For this review, take the finished solid that the model builds, in its own axes (mm). Round coordinates to 2 decimals unless told otherwise and drop trailing zeros. Loops run counter-clockwise (first coordinate to the right, second up) from the corner with the lowest first, then second, coordinate; pieces in that order, holes last. Notation, with made-up numbers: (39.5, 23.25) -> (78.5, 23.25) arc R13 ccw to (78.5, 34.25) -> close; hole circle Ø4 at (-34.75, 88.25). An arc over 180 degrees is marked (long way). Write each question's results on one line, items separated by ' | '.
```python
from build123d import *

# Parameters (mm, degrees)
SKETCH1_R           = 38.1
SKETCH1_R_2         = 29.21
BOSS_EXTRUDE1_DEPTH = 4
SKETCH2_R           = 1.75
CUT_EXTRUDE1_DEPTH  = 5
CUT_EXTRUDE2_DEPTH  = 2


with BuildPart() as part:
    # Sketch1 → Boss-Extrude1 (new body)
    with BuildSketch(Plane.XY):
        Circle(SKETCH1_R)
        Circle(SKETCH1_R_2, mode=Mode.SUBTRACT)
    extrude(amount=BOSS_EXTRUDE1_DEPTH)

    # Sketch2 → Cut-Extrude1 (cut, through all)
    with BuildSketch(Plane.XY.offset(4)):
        with Locations((0, 35.814)):
            Circle(SKETCH2_R)
        with Locations((17.907, 31.015833811)):
            Circle(SKETCH2_R)
        with Locations((31.015833811, 17.907)):
            Circle(SKETCH2_R)
        with Locations((35.814, 0)):
            Circle(SKETCH2_R)
        with Locations((31.015833811, -17.907)):
            Circle(SKETCH2_R)
        with Locations((17.907, -31.015833811)):
            Circle(SKETCH2_R)
        with Locations((0, -35.814)):
            Circle(SKETCH2_R)
        with Locations((-17.907, -31.015833811)):
            Circle(SKETCH2_R)
        with Locations((-31.015833811, -17.907)):
            Circle(SKETCH2_R)
        with Locations((-35.814, 0)):
            Circle(SKETCH2_R)
        with Locations((-31.015833811, 17.907)):
            Circle(SKETCH2_R)
        with Locations((-17.907, 31.015833811)):
            Circle(SKETCH2_R)
    extrude(amount=-CUT_EXTRUDE1_DEPTH, mode=Mode.SUBTRACT)

    # Sketch3 → Cut-Extrude2 (cut)
    with BuildSketch(Plane.XY.offset(4)):
        Polygon((-2.9, 37.989472226), (0, 39.162631561), (2.9, 37.989472226), (2.9, 34.139684219), (0, 32.465368439), (-2.9, 34.139684219), align=None)
        Polygon((16.483262442, 34.349848024), (19.581315781, 33.915833811), (21.506209784, 31.449848024), (19.581315781, 28.115833811), (16.232684219, 28.115833811), (14.558368439, 31.015833811), align=None)
        Polygon((31.449848024, 21.506209784), (33.915833811, 19.581315781), (34.349848024, 16.483262442), (31.015833811, 14.558368439), (28.115833811, 16.232684219), (28.115833811, 19.581315781), align=None)
        Polygon((37.989472226, 2.9), (39.162631561, 0), (37.989472226, -2.9), (34.139684219, -2.9), (32.465368439, 0), (34.139684219, 2.9), align=None)
        Polygon((34.349848024, -16.483262442), (33.915833811, -19.581315781), (31.449848024, -21.506209784), (28.115833811, -19.581315781), (28.115833811, -16.232684219), (31.015833811, -14.558368439), align=None)
        Polygon((21.506209784, -31.449848024), (19.581315781, -33.915833811), (16.483262442, -34.349848024), (14.558368439, -31.015833811), (16.232684219, -28.115833811), (19.581315781, -28.115833811), align=None)
        Polygon((2.9, -37.989472226), (0, -39.162631561), (-2.9, -37.989472226), (-2.9, -34.139684219), (0, -32.465368439), (2.9, -34.139684219), align=None)
        Polygon((-16.483262442, -34.349848024), (-19.581315781, -33.915833811), (-21.506209784, -31.449848024), (-19.581315781, -28.115833811), (-16.232684219, -28.115833811), (-14.558368439, -31.015833811), align=None)
        Polygon((-31.449848024, -21.506209784), (-33.915833811, -19.581315781), (-34.349848024, -16.483262442), (-31.015833811, -14.558368439), (-28.115833811, -16.232684219), (-28.115833811, -19.581315781), align=None)
        Polygon((-37.989472226, -2.9), (-39.162631561, 0), (-37.989472226, 2.9), (-34.139684219, 2.9), (-32.465368439, 0), (-34.139684219, -2.9), align=None)
        Polygon((-34.349848024, 16.483262442), (-33.915833811, 19.581315781), (-31.449848024, 21.506209784), (-28.115833811, 19.581315781), (-28.115833811, 16.232684219), (-31.015833811, 14.558368439), align=None)
        Polygon((-21.506209784, 31.449848024), (-19.581315781, 33.915833811), (-16.483262442, 34.349848024), (-14.558368439, 31.015833811), (-16.232684219, 28.115833811), (-19.581315781, 28.115833811), align=None)
    extrude(amount=-CUT_EXTRUDE2_DEPTH, mode=Mode.SUBTRACT)


solid = part.part
```
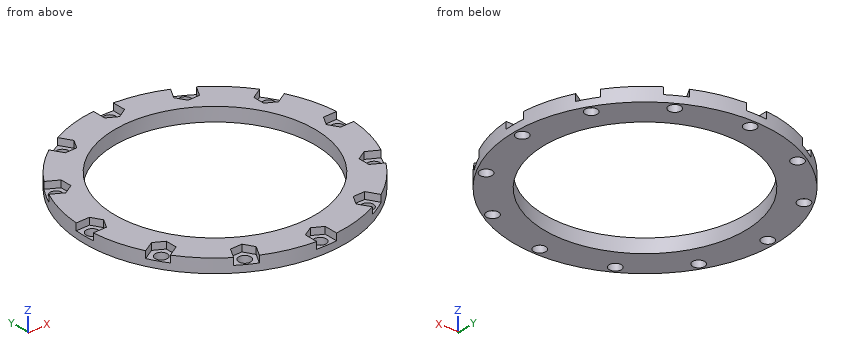
1. Consider section A-A (z = 0.95). Give the number of separate pieces and of enclosed holes in the cut face, plus the area to 3 significant figures.
Values found:
separate pieces: 1 | enclosed holes: 13 | area: 1,760 mm2
2. Consider section B-B (y = 13). State the section outline as (x, z) points, plus the area to 3 significant figures.
Values found:
outline: (-35.81, 0) -> (-26.16, 0) -> (-26.16, 4) -> (-35.81, 4) -> close; (26.16, 0) -> (35.81, 0) -> (35.81, 4) -> (26.16, 4) -> close | area: 77.2 mm2
3. Consider section C-C (x = 4). State the section outline as (y, z) points, plus the area to 3 significant figures.
Values found:
outline: (-37.89, 0) -> (-28.93, 0) -> (-28.93, 4) -> (-37.89, 4) -> close; (28.93, 0) -> (37.89, 0) -> (37.89, 4) -> (28.93, 4) -> close | area: 71.6 mm2
4. To check wall thickness, follow probe 1 along Y at (x, z) = (0, 1.45); probe 2 along X at (y, z) = (-32.5, 0.85); probe 3 along Y at (x, z) = (1.5, 1). State the ranges of each line that lie inside material, in increasing order.
Values found:
probe 1: y = -38.1 to -37.56, -34.06 to -29.21, 29.21 to 34.06, 37.56 to 38.1 | probe 2: x = -19.88 to -18.83, -16.98 to 16.98, 18.83 to 19.88 | probe 3: y = -38.07 to -36.72, -34.91 to -29.17, 29.17 to 34.91, 36.72 to 38.07
5. For pin 1 (2 mm diameter, centred on x = 18, z = 3.5, fed in from -Y); pin 2 (2 mm diameter, centred on x = -5.5, z = 1.5, fed in from +Y); pin 3 (5.5 mm diameter, centred on x = -17.91, y = 31.02, fed in from +Z), all flat-tipped, find the tip position at first contact; note any pin that passes through.
Values found:
pin 1: stops at y = -28.12 | pin 2: stops at y = 37.83 | pin 3: stops at z = 2
